Geometry check sheet. Reference: the model listing, model coordinates, mm. A direction names the side the tool comes from. Coordinates: 2 decimals unless noted, no trailing zeros. Order: outer loops, then holes, each group sorted by start corner. A loop starts at its lowest first (then second) coordinate and runs counter-clockwise, first axis right, second up.
```python
from build123d import *

# Parameters (mm, degrees)
F1_DEPTH = 470
F2_R     = 4
F3_DEPTH = 25
F4_R     = 7.5
F5_DEPTH = 11


with BuildPart() as f1:
    # F0 (on Front) → F1 (new body)
    with BuildSketch(Plane.XZ):
        with BuildLine():
            Line((0, 8), (0, 0))
            Line((0, 0), (28, 0))
            Line((28, 0), (28, 8))
            ThreePointArc((28, 8), (25, 11), (28, 14))
            Line((28, 14), (28, 19))
            ThreePointArc((28, 19), (25.87868, 19.87868), (25, 22))
            Line((25, 22), (3, 22))
            ThreePointArc((3, 22), (2.12132, 19.87868), (0, 19))
            Line((0, 19), (0, 14))
            ThreePointArc((0, 14), (3, 11), (0, 8))
        make_face()
    extrude(amount=F1_DEPTH)

    # F2 (on face) → F3 (cut)
    with BuildSketch(Plane.XY.offset(22)):
        with Locations((14, -45)):
            Circle(F2_R)
        with Locations((14, -125)):
            Circle(F2_R)
        with Locations((14, -205)):
            Circle(F2_R)
        with Locations((14, -285)):
            Circle(F2_R)
        with Locations((14, -365)):
            Circle(F2_R)
        with Locations((14, -445)):
            Circle(F2_R)
    extrude(amount=-F3_DEPTH, mode=Mode.SUBTRACT)

    # F4 (on face) → F5 (cut)
    with BuildSketch(Plane.XY.offset(22)):
        with Locations((14, -205)):
            Circle(F4_R)
        with Locations((14, -125)):
            Circle(F4_R)
        with Locations((14, -45)):
            Circle(F4_R)
        with Locations((14, -285)):
            Circle(F4_R)
        with Locations((14, -365)):
            Circle(F4_R)
        with Locations((14, -445)):
            Circle(F4_R)
    extrude(amount=-F5_DEPTH, mode=Mode.SUBTRACT)


solid = f1.part
```
Item 1: Sectioned sample at A-A (y = -445). Record the cut outline in (x, z), and give its area (3 significant figures).
Item 2: Thickness scan on line 1 along X through (y, z) = (-285, 14.5); line 2 along Z through (x, y) = (2.25, -390); line 3 along X through (y, z) = (-370.5, 12). Record the ranges inside material, lowest first.
Item 3: Sectioned sample at B-B (y = -58). Record the cut outline in (x, z).
Item 4: Release check for a two-part mould opening along Y. For faces 3 (the face through (14, -470, 11)), 4 (the face through (13.479, -121.034, 5.577)), 5 (the face through (14, -232, 22)) record: pulls with the +Y half, pulls with the -Y half, needs draft (parallel to the pull), parting line crosses it, or undercut.
Item 5: Tool access check on faces 1 (the face through (15.846, -368.549, 5.577)), 2 (the face through (12.37, -452.32, 16.58)). Record the directions out of +Z, -Z, +X, -X, +Y, -Y that give a thin tool (end or side, any length) a straight path to the whole face; none if there is none.
Item 6: Depth check by flat-ended pin: P1, Ø7.5, axis at x = 13, y = -42, coming from the +Z side; P2, Ø1.5, axis at y = -195.5, z = 12.5, coming from the -X side. Enter the tip coordinate at first touch or a pass-through.
Geometry check:
1. outline: (0, 0) - (10, 0) - (10, 11) - (6.5, 11) - (6.5, 22) - (3, 22) arc R3 cw to (0, 19) - (0, 14) arc R3 cw to (0, 8) - close; (18, 0) - (28, 0) - (28, 8) arc R3 cw to (28, 14) - (28, 19) arc R3 cw to (25, 22) - (21.5, 22) - (21.5, 11) - (18, 11) - close
1. area: 321 mm2
2. line 1: x = 0 to 6.5, 21.5 to 28
2. line 2: z = 0 to 9.02, 12.98 to 20.02
2. line 3: x = 2.83 to 8.9, 19.1 to 25.17
3. outline: (0, 0) - (28, 0) - (28, 8) arc R3 cw to (28, 14) - (28, 19) arc R3 cw to (25, 22) - (3, 22) arc R3 cw to (0, 19) - (0, 14) arc R3 cw to (0, 8) - close
4. face 3: pulls with the -Y half
4. face 4: undercut
4. face 5: needs draft
5. face 1: +Z, -Z
5. face 2: +Z
6. P1: stops at z = 11
6. P2: stops at x = 1.98
